from build123d import *

# Parameters (mm, degrees)
F1_DEPTH = 15.875


with BuildPart() as f1:
    # F0 (on Top) → F1 (new body)
    with BuildSketch(Plane.XY):
        Polygon((-114.410472, 425.45), (-444.5, 425.45), (-444.5, 406.4), (-495.284437, 406.4), (-495.284437, 139.7), (-444.5, 139.7), (-444.5, 120.65), (-114.410472, 120.65), (-114.410472, 139.7), (-81.119703, 139.7), (-57.579575, 116.159872), (-71.04996, 102.689488), (172.539488, -140.89996), (186.009872, -127.429575), (209.55, -150.969703), (209.55, -174.735472), (476.25, -174.735472), (476.25, -133.460472), (495.3, -133.460472), (495.3, 374.65), (476.25, 374.65), (476.25, 406.4), (425.45, 406.4), (425.45, 425.45), (-63.610472, 425.45), (-63.610472, 406.4), (-114.410472, 406.4), align=None)
    extrude(amount=F1_DEPTH)


solid = f1.part
Here's how the part is built. I have some questions about the finished solid (model axes, mm). A direction names the side the tool comes from. Round coordinates to 2 decimals unless told otherwise and drop trailing zeros. Write each loop counter-clockwise with the first axis right and the second up, starting at its lowest first coordinate (ties: lowest second). Pieces come first, ordered by that corner, then holes. Notation, with made-up numbers: (-11.5, 67) -> (31.5, 67) arc R27 ccw to (31.5, 104) -> close; hole circle Ø1 at (26.25, 22). An arc over 180 degrees is marked (long way). One line per item, written item: value.
1) Suppose I cut it at B-B on x = -171. List the corners of the cut face in (y, z) for me (3 decimals).
Filled sheet:
outline: (120.65, 0) -> (425.45, 0) -> (425.45, 15.875) -> (120.65, 15.875) -> close
2) If I drill on line 1 (Y direction, x = -204, z = 15); line 2 (Y direction, x = -91.5, z = 10.5); line 3 (X direction, y = 379, z = 11.75), over which ranges is the centre line in solid material (lowest first)? Write a range as [from, to].
Filled sheet:
line 1: y = [120.65, 425.45]
line 2: y = [139.7, 406.4]
line 3: x = [-495.28, 476.25]
3) Suppose I cut it at C-C on y = -117. List the corners of the cut face in (x, z) for me (3 decimals).
Filled sheet:
outline: (148.64, 0) -> (495.3, 0) -> (495.3, 15.875) -> (148.64, 15.875) -> close
4) I'm going to push flat-ended pins straight in: pin 1 Ø5 at (y, z) = (-144.5, 7) entering from +X; pin 2 Ø1.5 at (x, z) = (-8.5, 14) entering from -Y; pin 3 Ø8 at (y, z) = (132, 7) entering from -X. Where does each tip first touch, or does it pass through?
Filled sheet:
pin 1: stops at x = 476.25
pin 2: stops at y = 39.39
pin 3: stops at x = -444.5
5) Suppose I cut it at A-A on z = 6. List the corners of the cut face in (x, y) for me, plus the area to 3 significant figures.
Filled sheet:
outline: (-495.28, 139.7) -> (-444.5, 139.7) -> (-444.5, 120.65) -> (-114.41, 120.65) -> (-114.41, 139.7) -> (-81.12, 139.7) -> (-57.58, 116.16) -> (-71.05, 102.69) -> (172.54, -140.9) -> (186.01, -127.43) -> (209.55, -150.97) -> (209.55, -174.74) -> (476.25, -174.74) -> (476.25, -133.46) -> (495.3, -133.46) -> (495.3, 374.65) -> (476.25, 374.65) -> (476.25, 406.4) -> (425.45, 406.4) -> (425.45, 425.45) -> (-63.61, 425.45) -> (-63.61, 406.4) -> (-114.41, 406.4) -> (-114.41, 425.45) -> (-444.5, 425.45) -> (-444.5, 406.4) -> (-495.28, 406.4) -> close
area: 423,000 mm2
6) For faces 1 (the face through (49.04, -17.4, 7.83)), 2 (the face through (197.615, -139.035, 7.826)), 3 (the face through (-69.51, 128.09, 7.83)), which set-ups out of +Z, -Z, +X, -X, +Y, -Y let a thin tool reach every point of the face, with its end or its side?
Filled sheet:
face 1: +Z, -Z, -X, -Y
face 2: +Z, -Z, -Y
face 3: +Z, -Z
